from build123d import *

# Parameters (mm, degrees)
BOSS_EXTRUDE1_DEPTH         = 10
CUT_EXTRUDE1_DEPTH          = 67.21933252457322
CUT_EXTRUDE2_DEPTH          = 2
M3_TAPPED_HOLE1_D           = 2.5
M3_TAPPED_HOLE1_DEPTH       = 9
M3_TAPPED_HOLE1_CSINK_D     = 3.05
M3_TAPPED_HOLE1_CSINK_ANGLE = 90
M3_TAPPED_HOLE1_TIP         = 0.7510757737844503
SKETCH5_R                   = 2.4999999999999987
CUT_EXTRUDE3_DEPTH          = 44.18564576337837
SKETCH6_R                   = 4
CUT_EXTRUDE4_DEPTH          = 53.191953402799555
CHAMFER1_SIZE               = 1
HOLE1_START                 = 2
HOLE1_OUTLINE_R             = 2
HOLE1_DEPTH                 = 28
HOLE1_START_2               = -16.200329062
HOLE1_2_OUTLINE_R           = 1.25
HOLE1_2_DEPTH               = 18.200329062
CUT_EXTRUDE5_REACH          = 54.192
CUT_EXTRUDE5_END_RADIUS     = 7
SKETCH9_R                   = 1.6000000000000005
M4_TAPPED_HOLE1_REACH       = 68.219
M4_TAPPED_HOLE1_BORE_R      = 1.65
CUT_EXTRUDE6_REACH          = 68.219
CUT_EXTRUDE6_END_RADIUS     = 2.4999999999999987
SKETCH12_R                  = 1.2499999999999991


# Read off the part's stored shape, not the designer's step: Hole1
with BuildPart() as part:
    # Sketch1 → Boss-Extrude1 (new, symmetric)
    with BuildSketch(Plane.XY):
        Polygon((0, 0), (-19.000000000000004, -3.04e-15), (-19, 32), (8.999999999999991, 32), (21, -5.9999999999999964), (21, -29.999999999999996), (3.47e-15, -30), align=None)
    extrude(amount=BOSS_EXTRUDE1_DEPTH, both=True)

    # Sketch2 → Cut-Extrude1 (cut, through all)
    with BuildSketch(Plane(origin=(0, 32, 0), x_dir=(1, 0, 0), z_dir=(0, 1, 0))):
        with BuildLine():
            ThreePointArc((-2.2917960675006315, 2.000000000000001), (-10.010587075047079, 6.926666858146693), (-16, -2.25e-15))
            Line((-16, 0), (-2, 0))
            ThreePointArc((-2, 0), (-2.0733331418533067, 1.0105870750470785), (-2.2917960675006315, 2.000000000000001))
        make_face()
        with BuildLine():
            Line((-2, 0), (-16, 0))
            ThreePointArc((-16, 8.6e-16), (-10.01058707504708, -6.926666858146693), (-2.2917960675006324, -2.0000000000000036))
            ThreePointArc((-2.2917960675006324, -2.0000000000000036), (-2.0733331418533067, -1.0105870750470807), (-2, -1.71e-15))
        make_face()
    extrude(amount=-CUT_EXTRUDE1_DEPTH, mode=Mode.SUBTRACT)

    # Sketch2<3> → Cut-Extrude2 (cut)
    with BuildSketch(Plane(origin=(0, 32, 0), x_dir=(1, 0, 0), z_dir=(0, 1, 0))):
        with BuildLine():
            ThreePointArc((5.000000000000001, 2.0000000000000004), (3.585786437626906, 1.4142135623730954), (3.0000000000000004, 2.4e-16))
            Line((3, 0), (7, 0))
            ThreePointArc((7.000000000000002, 0), (6.414213562373096, 1.4142135623730951), (5.000000000000001, 2.0000000000000004))
        make_face()
        with BuildLine():
            Line((7, 0), (3, 0))
            ThreePointArc((3.0000000000000004, 2.4e-16), (3.585786437626905, -1.4142135623730951), (5.000000000000001, -2.0000000000000004))
            ThreePointArc((5.000000000000001, -2.0000000000000004), (6.414213562373096, -1.4142135623730956), (7.000000000000002, -4.9e-16))
        make_face()
        with BuildLine():
            Line((3, 0), (-2, 0))
            ThreePointArc((-2, -1.71e-15), (-2.0733331418533067, -1.0105870750470807), (-2.2917960675006324, -2.0000000000000036))
            Line((-2.2917960675006315, -2.0000000000000013), (5.000000000000001, -2.0000000000000004))
            ThreePointArc((5.000000000000001, -2.0000000000000004), (3.585786437626905, -1.4142135623730951), (3.0000000000000004, 2.4e-16))
        make_face()
        with BuildLine():
            ThreePointArc((-2.2917960675006315, 2.000000000000001), (-2.0733331418533067, 1.0105870750470785), (-2, 0))
            Line((-2, 0), (3, 0))
            ThreePointArc((3.0000000000000004, 2.4e-16), (3.585786437626906, 1.4142135623730954), (5.000000000000001, 2.0000000000000004))
            Line((5.000000000000001, 2.0000000000000004), (-2.2917960675006315, 2.0000000000000013))
        make_face()
    extrude(amount=-CUT_EXTRUDE2_DEPTH, mode=Mode.SUBTRACT)

    # M3 Tapped Hole1
    with Locations(Plane(origin=(0, 32, 0), x_dir=(1, 0, 0), z_dir=(0, 1, 0))):
        with Locations((-16.363887926, 7), (-16.363887926, -7), (5, -7), (5, 7)):
            CounterSinkHole(M3_TAPPED_HOLE1_D / 2, M3_TAPPED_HOLE1_CSINK_D / 2, depth=M3_TAPPED_HOLE1_DEPTH, counter_sink_angle=M3_TAPPED_HOLE1_CSINK_ANGLE)
            with Locations((0, 0, -(M3_TAPPED_HOLE1_DEPTH + M3_TAPPED_HOLE1_TIP / 2))):  # 118° drill point
                Cone(0, M3_TAPPED_HOLE1_D / 2, M3_TAPPED_HOLE1_TIP, mode=Mode.SUBTRACT)

    # Sketch5 → Cut-Extrude3 (cut, through all)
    with BuildSketch(Plane.XY.offset(10)):
        with Locations((13.000000000000002, -9.999999999999998)):
            Circle(SKETCH5_R)
    extrude(amount=-CUT_EXTRUDE3_DEPTH, mode=Mode.SUBTRACT)

    # Sketch6 → Cut-Extrude4 (cut, through all)
    with BuildSketch(Plane(origin=(21, 0, 0), x_dir=(0, 0, -1), z_dir=(1, 0, 0))):
        with Locations((0, -19.999999999999996)):
            Circle(SKETCH6_R)
    extrude(amount=-CUT_EXTRUDE4_DEPTH, mode=Mode.SUBTRACT)

    # Chamfer1
    chamfer1_edges = [part.edges().sort_by_distance(p)[0] for p in [
        (21, -19.999999999999996, 4),
    ]]
    chamfer(chamfer1_edges, length=CHAMFER1_SIZE)

    # Hole1 outline → Hole1 (cut)
    with BuildSketch(Plane(origin=(0, 0, 0), x_dir=(1, 0, 0), z_dir=(0, 1, 0)).offset(HOLE1_START)):
        with Locations((5, 0)):
            Circle(HOLE1_OUTLINE_R)
    extrude(amount=HOLE1_DEPTH, mode=Mode.SUBTRACT)

    # Hole1 2 outline → Hole1 2 (cut)
    with BuildSketch(Plane(origin=(0, 0, 0), x_dir=(1, 0, 0), z_dir=(0, 1, 0)).offset(HOLE1_START_2)):
        with Locations((5, 0)):
            Circle(HOLE1_2_OUTLINE_R)
    extrude(amount=HOLE1_2_DEPTH, mode=Mode.SUBTRACT)

    # Cut-Extrude5: up to this cylinder (the profile starts outside it)
    cut_extrude5_end = Plane(origin=(-9, 15, 0), z_dir=(0, 1, 0)) * Cylinder(CUT_EXTRUDE5_END_RADIUS, 123.384, mode=Mode.PRIVATE)
    # Sketch9 → Cut-Extrude5 (cut, up to the surface)
    with BuildSketch(Plane.ZY.offset(19.000000000000004), mode=Mode.PRIVATE) as cut_extrude5_sk1:
        with Locations(Location((-2.999999999999998, 15, 0), (0, 0, 270))):
            Circle(SKETCH9_R)
    cut_extrude5_tool1 = extrude(cut_extrude5_sk1.sketch, amount=-CUT_EXTRUDE5_REACH, mode=Mode.PRIVATE) - cut_extrude5_end
    add(cut_extrude5_tool1.solids().sort_by_distance((-19, 15, -3))[0], mode=Mode.SUBTRACT)
    # Sketch9 → Cut-Extrude5 (cut, up to the surface)
    with BuildSketch(Plane.ZY.offset(19.000000000000004), mode=Mode.PRIVATE) as cut_extrude5_sk2:
        with Locations(Location((3.000000000000002, 15, 0), (0, 0, 270))):
            Circle(SKETCH9_R)
    cut_extrude5_tool2 = extrude(cut_extrude5_sk2.sketch, amount=-CUT_EXTRUDE5_REACH, mode=Mode.PRIVATE) - cut_extrude5_end
    add(cut_extrude5_tool2.solids().sort_by_distance((-19, 15, 3))[0], mode=Mode.SUBTRACT)

    # M4 Tapped Hole1 bore → M4 Tapped Hole1 (cut, up to next)
    with BuildSketch(Plane(origin=(4.96e-15, -30, 0), x_dir=(-1, -1.7e-16, 0), z_dir=(1.7e-16, -1, 0)), mode=Mode.PRIVATE) as m4_tapped_hole1_sk1:
        with Locations((-13, 0)):
            Circle(M4_TAPPED_HOLE1_BORE_R)
    m4_tapped_hole1_tool1 = extrude(m4_tapped_hole1_sk1.sketch, amount=-M4_TAPPED_HOLE1_REACH, mode=Mode.PRIVATE) & part.part
    # M4 Tapped Hole1 bore → M4 Tapped Hole1 (cut, up to next)
    with BuildSketch(Plane(origin=(4.96e-15, -30, 0), x_dir=(-1, -1.7e-16, 0), z_dir=(1.7e-16, -1, 0)), mode=Mode.PRIVATE) as m4_tapped_hole1_sk2:
        with Locations((-5, 0)):
            Circle(M4_TAPPED_HOLE1_BORE_R)
    m4_tapped_hole1_tool2 = extrude(m4_tapped_hole1_sk2.sketch, amount=-M4_TAPPED_HOLE1_REACH, mode=Mode.PRIVATE) & part.part
    add(m4_tapped_hole1_tool1.solids().sort_by_distance((13, -30, 0))[0], mode=Mode.SUBTRACT)
    add(m4_tapped_hole1_tool2.solids().sort_by_distance((5, -30, 0))[0], mode=Mode.SUBTRACT)

    # Cut-Extrude6: up to this cylinder (the profile starts outside it)
    cut_extrude6_end = Plane(origin=(13.000000000000002, -9.999999999999998, 0), z_dir=(0, 0, 1)) * Cylinder(CUT_EXTRUDE6_END_RADIUS, 142.438, mode=Mode.PRIVATE)
    # Sketch12 → Cut-Extrude6 (cut, up to the surface)
    with BuildSketch(Plane.XZ.offset(30), mode=Mode.PRIVATE) as cut_extrude6_sk1:
        with Locations((12.999999999999998, 0)):
            Circle(SKETCH12_R)
    cut_extrude6_tool1 = extrude(cut_extrude6_sk1.sketch, amount=-CUT_EXTRUDE6_REACH, mode=Mode.PRIVATE) - cut_extrude6_end
    add(cut_extrude6_tool1.solids().sort_by_distance((13, -30, 0))[0], mode=Mode.SUBTRACT)


solid = part.part
Verification items for the finished model (mm, model axes). A direction names the side the tool comes from. Round coordinates to 2 decimals unless told otherwise and drop trailing zeros. Loops run counter-clockwise (first coordinate to the right, second up) from the corner with the lowest first, then second, coordinate; pieces in that order, holes last. Notation, with made-up numbers: (-6, 29.5) - (15, 29.5) arc R21 ccw to (15, 62.5) - close; hole circle Ø7 at (67, 48). An arc over 180 degrees is marked (long way). Use a Markdown table: item, result. Add a question column.
1. Section check B-B, the plane x = -9. Record the boundary of the cut face in (y, z).
2. Section check C-C, the plane y = -20. Record the boundary of the cut face in (x, z).
3. Section check A-A, the plane y = -10. Record the boundary of the cut face in (x, z).
4. Release check for a two-part mould opening along X. For faces 1 (the face through (1, 1, -10)), 2 (the face through (-16.16, 22.38, 7.08)), 3 (the face through (-19, 16, 0)) record: released by +X, released by -X, zero draft, split by the parting line, or undercut.
5. Thickness scan on probe 1 along Z at (x, y) = (5, 26); probe 2 along Z at (x, y) = (-5, 10); probe 3 along X at (y, z) = (-9.25, 0). Record the ranges inside material, lowest first. Write a range as [from, to].
6. Gauge pin test, flat ends, axial feed: pin 1 (3 mm diameter, centred on x = -16.36, z = 7, fed in from -Y); pin 2 (4 mm diameter, centred on y = 15, z = 3, fed in from +X); pin 3 (3 mm diameter, centred on y = 15, z = -3, fed in from +X). Record the tip position at first contact, or that the pin passes through.
7. Section check D-D, the plane z = 3. Give the number of separate pieces and of enclosed holes in the cut face, plus the area to 3 significant figures.
8. Access from +Z, -Z, +X, -X, +Y, -Y to the whole of each face (thin tool, end or side, straight path). Record for faces 4 (the face through (-16, 0, 2)), 5 (the face through (21, -15, 2)), 6 (the face through (0, 30, 0)).
Checks:
| question | item | result |
|---|---|---|
| 1 | outline | (0, -10) - (32, -10) - (32, -7) - (0, -7) - close; (0, 7) - (32, 7) - (32, 10) - (0, 10) - close |
| 2 | outline | (0, -10) - (21, -10) - (21, -5) - (20, -4) - (0, -4) - close; (0, 4) - (20, 4) - (21, 5) - (21, 10) - (0, 10) - close |
| 3 | outline | (0, -10) - (10.5, -10) - (10.5, 10) - (0, 10) - close; (15.5, -10) - (21, -10) - (21, 10) - (15.5, 10) - close; hole circle Ø2.5 at (5, 0) |
| 4 | face 1 | zero draft |
| 4 | face 2 | undercut |
| 4 | face 3 | released by -X |
| 5 | probe 1 | z = [-10, -8.25], [-5.75, -2], [2, 5.75], [8.25, 10] |
| 5 | probe 2 | z = [-10, -5.74], [5.74, 10] |
| 5 | probe 3 | x = [0, 3.75], [6.25, 10.62], [15.38, 21] |
| 6 | pin 1 | stops at y = 0 |
| 6 | pin 2 | stops at x = 15 |
| 6 | pin 3 | stops at x = 14.84 |
| 7 | separate pieces | 4 |
| 7 | enclosed holes | 1 |
| 7 | area | 1,130 mm^2 |
| 8 | face 4 | +Z, -Z, -X, -Y |
| 8 | face 5 | +Z, -Z, +X, +Y, -Y |
| 8 | face 6 | +Y |
